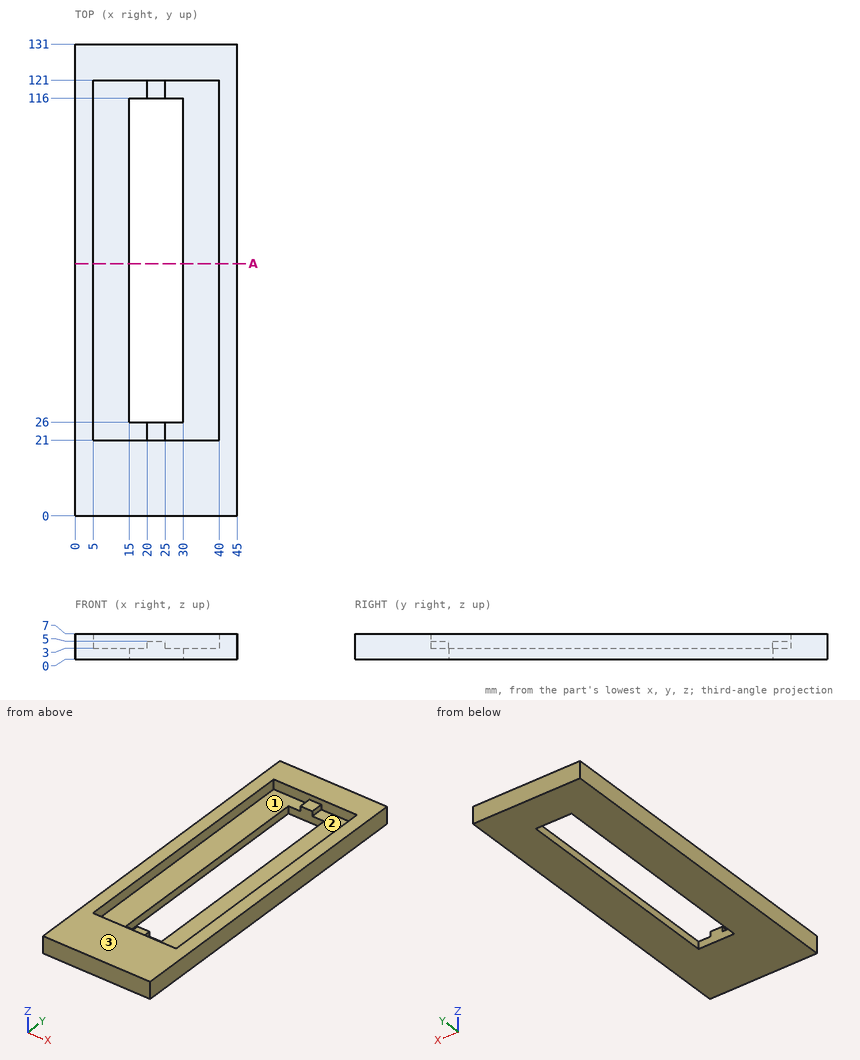
Could you check a few things on this drawing? It's one solid part, dimensions in mm from its lowest x, y, z. Coordinates: 2 decimals unless noted, no trailing zeros. Loops run counter-clockwise (first coordinate to the right, second up) from the corner with the lowest first, then second, coordinate; pieces in that order, holes last.
1. Imagine slicing it at A-A (y = 70). Please give me the cut outline in (x, z), and give its area (3 significant figures).
2. For P1, Ø2.5, axis at x = 23, y = 22.5, coming from the +Z side; P2, Ø16.5, axis at x = 29.5, y = 47.5, coming from the +Z side, each with a flat end and sliding along its axis, tell me the tip position at first contact or that it passes through.
3. We'd pull the mould along X, two halves only. Please class the marked faces 1, 2 and 3: released by +X, released by -X, zero draft, split by the parting line, or undercut.
4. I need wall thicknesses on L1, parallel to X at y = 118.5, z = 3.75; L2, parallel to Y at x = 8.5, z = 3.25; L3, parallel to X at y = 34.5, z = 6. Which ranges of each line are inside material? Lowest first, please.
Computed values:
1. outline: (0, 0) - (15, 0) - (15, 3) - (5, 3) - (5, 7) - (0, 7) - close; (30, 0) - (45, 0) - (45, 7) - (40, 7) - (40, 3) - (30, 3) - close
1. area: 130 mm2
2. P1: stops at z = 5
2. P2: stops at z = 3
3. face 1: undercut
3. face 2: undercut
3. face 3: zero draft
4. L1: x = 0 to 5, 20 to 25, 40 to 45
4. L2: y = 0 to 21, 121 to 131
4. L3: x = 0 to 5, 40 to 45
